from build123d import *

# Parameters (mm, degrees)
F1_DEPTH = 200


with BuildPart() as f1:
    # F0 (on Front) → F1 (new body)
    with BuildSketch(Plane.XZ):
        with BuildLine():
            ThreePointArc((27.5, 25.5), (26.914214, 26.914214), (25.5, 27.5))
            Line((25.5, 27.5), (-25.5, 27.5))
            ThreePointArc((-25.5, 27.5), (-26.914214, 26.914214), (-27.5, 25.5))
            Line((-27.5, 25.5), (-27.5, -25.5))
            ThreePointArc((-27.5, -25.5), (-26.914214, -26.914214), (-25.5, -27.5))
            Line((-25.5, -27.5), (25.5, -27.5))
            ThreePointArc((25.5, -27.5), (26.914214, -26.914214), (27.5, -25.5))
            Line((27.5, -25.5), (27.5, 25.5))
        make_face()
        with BuildLine():
            Line((-23, 25), (23, 25))
            ThreePointArc((23, 25), (24.414214, 24.414214), (25, 23))
            Line((25, 23), (25, -23))
            ThreePointArc((25, -23), (24.414214, -24.414214), (23, -25))
            Line((23, -25), (-23, -25))
            ThreePointArc((-23, -25), (-24.414214, -24.414214), (-25, -23))
            Line((-25, -23), (-25, 23))
            ThreePointArc((-25, 23), (-24.414214, 24.414214), (-23, 25))
        make_face(mode=Mode.SUBTRACT)
    extrude(amount=-F1_DEPTH)


solid = f1.part
The model under review builds one solid part; all positions refer to its coordinate system, in mm. A direction names the side the tool comes from. Give positions to 0.01 mm unless a question says otherwise; leave off trailing zeros. Loops run counter-clockwise (first coordinate to the right, second up) from the corner with the lowest first, then second, coordinate; pieces in that order, holes last. Notation, with made-up numbers: (61, 15.5) -> (72, 15.5) arc R19 cw to (72, 39.5) -> close; hole circle Ø6 at (55, 64.5). An arc over 180 degrees is marked (long way). Answer as a JSON object with one key per item and string values. Group by question number.
Q1. Take a section at C-C (y = 107). Write out the cut boundary in (x, z), plus the area to 3 significant figures.
Q2. Take a section at A-A (z = 18). Write out the cut boundary in (x, y), plus the area to 3 significant figures.
Q3. Draft analysis for pull direction Z (two halves, no side actions). For faces 3 (the flat face through (-27.5, 99, 0)), 4 (the flat face through (0, 99, -27.5)), 5 (the flat face through (0, 99, -25)), state which applies: pulls with the +Z half, pulls with the -Z half, needs draft (parallel to the pull), parting line crosses it, or undercut.
Q4. Tool access review of faces 1 (the flat face through (-27, 0, 0)), 2 (the flat face through (25, 99, 0)): name each direction out of +Z, -Z, +X, -X, +Y, -Y from which nothing blocks a thin tool from reaching the whole face with its end or side.
Q5. Wall thickness on line 1 along Z through (x, y) = (-9, 168.5); line 2 along Z through (x, y) = (-24, 174.5): over which ranges is each line inside the solid? List them lowest first.
Q6. Take a section at B-B (x = -21). Write out the cut boundary in (y, z), plus the area to 3 significant figures.
Answer below:
{
 "1": {"outline": "(-27.5, -25.5) arc R2 ccw to (-25.5, -27.5) -> (25.5, -27.5) arc R2 ccw to (27.5, -25.5) -> (27.5, 25.5) arc R2 ccw to (25.5, 27.5) -> (-25.5, 27.5) arc R2 ccw to (-27.5, 25.5) -> close; hole (-25, -23) arc R2 ccw to (-23, -25) -> (23, -25) arc R2 ccw to (25, -23) -> (25, 23) arc R2 ccw to (23, 25) -> (-23, 25) arc R2 ccw to (-25, 23) -> close", "area": "525 mm2"},
 "2": {"outline": "(-27.5, 0) -> (-25, 0) -> (-25, 200) -> (-27.5, 200) -> close; (25, 0) -> (27.5, 0) -> (27.5, 200) -> (25, 200) -> close", "area": "1,000 mm2"},
 "3": {"face 3": "needs draft", "face 4": "pulls with the -Z half", "face 5": "undercut"},
 "4": {"face 1": "+Z, -Z, +X, -X, -Y", "face 2": "+Y, -Y"},
 "5": {"line 1": "z = -27.5 to -25, 25 to 27.5", "line 2": "z = -27.5 to -24.73, 24.73 to 27.5"},
 "6": {"outline": "(0, -27.5) -> (200, -27.5) -> (200, -25) -> (0, -25) -> close; (0, 25) -> (200, 25) -> (200, 27.5) -> (0, 27.5) -> close", "area": "1,000 mm2"}
}
